from build123d import *

# Parameters (mm, degrees)
BOSS_EXTRUDE2_DEPTH = 27
CUT_EXTRUDE3_DEPTH  = 25
SKETCH5_R           = 10
CUT_EXTRUDE4_DEPTH  = 2
SKETCH6_W           = 6
SKETCH6_H           = 4
BOSS_EXTRUDE3_DEPTH = 27
SKETCH7_R           = 1.5
CUT_EXTRUDE5_DEPTH  = 27
SKETCH15_W          = 17
SKETCH15_H          = 12
CUT_EXTRUDE6_DEPTH  = 24
FILLET1_R           = 2
CUT_EXTRUDE10_DEPTH = 25
SKETCH21_R          = 2.5
CUT_EXTRUDE11_DEPTH = 10


with BuildPart() as part:
    # Sketch1 → Boss-Extrude2 (new body)
    with BuildSketch(Plane(origin=(0, 0, 0), x_dir=(1, 0, 0), z_dir=(0, 1, 0))):
        with BuildLine():
            Line((8.5, 11.734748557), (8.5, 25.734748557))
            Line((8.5, 25.734748557), (-8.5, 25.734748557))
            Line((-8.5, 25.734748557), (-8.5, 11.734748557))
            Line((-8.5, 11.734748557), (-36.552303323, 11.734748557))
            ThreePointArc((-36.552303323, 11.734748557), (-43.25, -3.515251443), (-36.552303323, -18.765251443))
            Line((-36.552303323, -18.765251443), (-8.5, -18.765251443))
            Line((-8.5, -18.765251443), (-8.5, -30.765251443))
            Line((-8.5, -30.765251443), (8.5, -30.765251443))
            Line((8.5, -30.765251443), (8.5, -18.765251443))
            Line((8.5, -18.765251443), (36.552303323, -18.765251443))
            ThreePointArc((36.552303323, -18.765251443), (43.25, -3.515251443), (36.552303323, 11.734748557))
            Line((36.552303323, 11.734748557), (8.5, 11.734748557))
        make_face()
    extrude(amount=BOSS_EXTRUDE2_DEPTH)

    # Sketch4 → Cut-Extrude3 (cut)
    with BuildSketch(Plane(origin=(0, 27, 0), x_dir=(1, 0, 0), z_dir=(0, 1, 0))):
        with BuildLine():
            Line((6.5, 9.734748557), (35.75, 9.734748557))
            ThreePointArc((35.75, 9.734748557), (41.25, -3.515251443), (35.75, -16.765251443))
            Line((35.75, -16.765251443), (-35.75, -16.765251443))
            ThreePointArc((-35.75, -16.765251443), (-41.25, -3.515251443), (-35.75, 9.734748557))
            Line((-35.75, 9.734748557), (-6.5, 9.734748557))
            Line((-6.5, 9.734748557), (-6.5, 11.734748557))
            Line((-6.5, 11.734748557), (6.5, 11.734748557))
            Line((6.5, 11.734748557), (6.5, 9.734748557))
        make_face()
    extrude(amount=-CUT_EXTRUDE3_DEPTH, mode=Mode.SUBTRACT)

    # Sketch5 → Cut-Extrude4 (cut)
    with BuildSketch(Plane.XZ):
        with Locations(Location((0, 3.515251443, 0), (0, 0, 270))):
            Circle(SKETCH5_R)
    extrude(amount=-CUT_EXTRUDE4_DEPTH, mode=Mode.SUBTRACT)

    # Sketch6 → Boss-Extrude3 (add)
    with BuildSketch(Plane(origin=(0, 27, 0), x_dir=(1, 0, 0), z_dir=(0, 1, 0))):
        with Locations((-33.552303323, 13.734748557)):
            Rectangle(SKETCH6_W, SKETCH6_H)
        with Locations((-33.552303323, -20.765251443)):
            Rectangle(SKETCH6_W, SKETCH6_H)
        with Locations((33.552303323, -20.765251443)):
            Rectangle(SKETCH6_W, SKETCH6_H)
        with Locations((33.552303323, 13.734748557)):
            Rectangle(SKETCH6_W, SKETCH6_H)
    extrude(amount=-BOSS_EXTRUDE3_DEPTH)

    # Sketch7 → Cut-Extrude5 (cut)
    with BuildSketch(Plane(origin=(0, 27, 0), x_dir=(1, 0, 0), z_dir=(0, 1, 0))):
        with Locations(Location((-33.552303323, 12.734748557, 0), (0, 0, 270))):
            Circle(SKETCH7_R)
        with Locations(Location((-33.552303323, -19.765251443, 0), (0, 0, 90))):
            Circle(SKETCH7_R)
        with Locations(Location((33.552303323, -19.765251443, 0), (0, 0, 270))):
            Circle(SKETCH7_R)
        with Locations(Location((33.552303323, 12.734748557, 0), (0, 0, 90))):
            Circle(SKETCH7_R)
    extrude(amount=-CUT_EXTRUDE5_DEPTH, mode=Mode.SUBTRACT)

    # Sketch15 → Cut-Extrude6 (cut)
    with BuildSketch(Plane.XZ):
        with Locations((0, -19.734748557)):
            Rectangle(SKETCH15_W, SKETCH15_H)
        with Locations((0, 24.765251443)):
            Rectangle(SKETCH15_W, SKETCH15_H)
    extrude(amount=-CUT_EXTRUDE6_DEPTH, mode=Mode.SUBTRACT)

    # Fillet1
    fillet1_edges = [part.edges().sort_by_distance(p)[0] for p in [
        (36.552303323, 13.5, -15.734748557),
        (30.552303323, 13.5, -15.734748557),
        (-30.552303323, 13.5, -15.734748557),
        (-36.552303323, 13.5, -15.734748557),
        (-36.552303323, 13.5, 22.765251443),
        (-30.552303323, 13.5, 22.765251443),
        (30.552303323, 13.5, 22.765251443),
        (36.552303323, 13.5, 22.765251443),
    ]]
    fillet(fillet1_edges, radius=FILLET1_R)

    # Sketch20 → Cut-Extrude10 (cut)
    with BuildSketch(Plane(origin=(0, 27, 0), x_dir=(1, 0, 0), z_dir=(0, 1, 0))):
        with BuildLine():
            Line((6.5, 9.884748557), (-6.5, 9.884748557))
            Line((-6.5, 9.884748557), (-35.811855186, 9.884748557))
            ThreePointArc((-35.811855186, 9.884748557), (-41.4, -3.515251443), (-35.811855186, -16.915251443))
            Line((-35.811855186, -16.915251443), (35.811855186, -16.915251443))
            ThreePointArc((35.811855186, -16.915251443), (41.4, -3.515251443), (35.811855186, 9.884748557))
            Line((35.811855186, 9.884748557), (6.5, 9.884748557))
        make_face()
        with BuildLine():
            Line((35.75, 9.734748557), (6.5, 9.734748557))
            Line((6.5, 9.734748557), (-6.5, 9.734748557))
            Line((-6.5, 9.734748557), (-35.75, 9.734748557))
            ThreePointArc((-35.75, 9.734748557), (-41.25, -3.515251443), (-35.75, -16.765251443))
            Line((-35.75, -16.765251443), (35.75, -16.765251443))
            ThreePointArc((35.75, -16.765251443), (41.25, -3.515251443), (35.75, 9.734748557))
        make_face(mode=Mode.SUBTRACT)
    extrude(amount=-CUT_EXTRUDE10_DEPTH, mode=Mode.SUBTRACT)

    # Sketch21 → Cut-Extrude11 (cut)
    with BuildSketch(Plane(origin=(0, 27, 0), x_dir=(1, 0, 0), z_dir=(0, 1, 0))):
        with Locations(Location((0, 18.734748557, 0), (0, 0, 270))):
            Circle(SKETCH21_R)
        with Locations(Location((0, -24.765251443, 0), (0, 0, 270))):
            Circle(SKETCH21_R)
    extrude(amount=-CUT_EXTRUDE11_DEPTH, mode=Mode.SUBTRACT)


solid = part.part
Geometry check sheet. Reference: the model listing, model coordinates, mm. A direction names the side the tool comes from. Coordinates: 2 decimals unless noted, no trailing zeros. Order: outer loops, then holes, each group sorted by start corner. A loop starts at its lowest first (then second) coordinate and runs counter-clockwise, first axis right, second up. Notation, with made-up numbers: (-16.75, 88) - (-0.75, 88) arc R22 cw to (-0.75, 116) - close; hole circle Ø6 at (33.5, -25). An arc over 180 degrees is marked (long way). Answer in a Markdown table with one row per item. Add a question column.
1) Cross-section at C-C, the plane z = -8. Record the cut outline in (x, y), then the cut area to 3 significant figures.
2) Cross-section at B-B, the plane x = 13.5. Record the cut outline in (y, z).
3) Cross-section at D-D, the plane y = 25. State how many separate pieces and enclosed holes the cut face has, then the cut area to 3 significant figures.
4) Cross-section at A-A, the plane x = 0. Record the cut outline in (y, z).
5) Gauge pin test, flat ends, axial feed: P1, Ø8, axis at x = -19, y = 16, coming from the +Z side; P2, Ø1.5, axis at y = 25.5, z = 24, coming from the +X side; P3, Ø3.5, axis at x = 0, z = -21.5, coming from the -Y side. Record the tip position at first contact, or that the pin passes through.
6) Release check for a two-part mould opening along X. For faces 1 (the flat face through (30.552, 14, -13)), 2 (the flat face through (36.552, 14, -13)), 3 (the cylindrical face through (-35.951, 13.311, 22.195)) record: +X half, -X half, draft (parallel to the pull), parting line (faces both ways), or undercut.
7) Set-up check for faces 4 (the flat face through (-6.5, 15, -11)), 5 (the flat face through (-2, 24, -21)), 6 (the flat face through (-36.552, 14, 20)): record each of +Z, -Z, +X, -X, +Y, -Y from which the full face is reachable in a straight line by a thin tool's end or side.
8) Material ranges on line 1 along Z through (x, y) = (-14.5, 25.5); line 2 along Z through (x, y) = (1.5, 23.5); line 3 along X through (y, z) = (22.75, 19.5), recorded low to high. Write a range as [from, to].
Check result:
| question | item | result |
|---|---|---|
| 1 | outline | (-39.75, 0) - (39.75, 0) - (39.75, 27) - (37.48, 27) - (37.48, 2) - (-37.48, 2) - (-37.48, 27) - (-39.75, 27) - close |
| 1 | area | 273 mm² |
| 2 | outline | (0, -11.73) - (27, -11.73) - (27, -9.88) - (2, -9.88) - (2, 16.92) - (27, 16.92) - (27, 18.77) - (0, 18.77) - close |
| 3 | separate pieces | 1 |
| 3 | enclosed holes | 7 |
| 3 | area | 826 mm² |
| 4 | outline | (0, -13.73) - (24, -13.73) - (24, -16.23) - (27, -16.23) - (27, -11.73) - (2, -11.73) - (2, -6.48) - (0, -6.48) - close; (0, 13.52) - (2, 13.52) - (2, 16.92) - (27, 16.92) - (27, 22.27) - (24, 22.27) - (24, 18.77) - (0, 18.77) - close; (24, -25.73) - (27, -25.73) - (27, -21.23) - (24, -21.23) - close; (24, 27.27) - (27, 27.27) - (27, 30.77) - (24, 30.77) - close |
| 5 | P1 | stops at z = 18.77 |
| 5 | P2 | stops at x = 8.5 |
| 5 | P3 | stops at y = 24 |
| 6 | face 1 | undercut |
| 6 | face 2 | +X half |
| 6 | face 3 | -X half |
| 7 | face 4 | +Y |
| 7 | face 5 | -Z, -Y |
| 7 | face 6 | +Z, -X, +Y, -Y |
| 8 | line 1 | z = [-11.73, -9.88], [16.92, 18.77] |
| 8 | line 2 | z = [-13.73, -11.73], [16.92, 18.77] |
| 8 | line 3 | x = [-36.55, -35.03], [-32.08, -30.55], [30.55, 32.08], [35.03, 36.55] |
